Geometry check sheet. Reference: the model listing, model coordinates, mm. A direction names the side the tool comes from. Round coordinates to 2 decimals unless told otherwise and drop trailing zeros. Write each loop counter-clockwise with the first axis right and the second up, starting at its lowest first coordinate (ties: lowest second). Pieces come first, ordered by that corner, then holes. Notation, with made-up numbers: (67, 86) -> (115, 86) arc R25 ccw to (115, 121) -> close; hole circle Ø3 at (-16, 69). An arc over 180 degrees is marked (long way). One line per question, with ' | ' between items.
```python
from build123d import *

# Parameters (mm, degrees)
SKETCH2_R                = 7
BOSS_EXTRUDE1_DEPTH      = 20
BOSS_EXTRUDE1_2_DEPTH    = 20
BOSS_EXTRUDE4_DEPTH      = 25
BOSS_EXTRUDE4_DEPTH_BACK = 25
BOSS_EXTRUDE5_REACH      = 52
SKETCH5_W                = 40
SKETCH5_H                = 30
SKETCH5_W_2              = 30
SKETCH5_H_2              = 20
SKETCH6_R                = 7.5
CUT_EXTRUDE1_DEPTH       = 51


with BuildPart() as part:
    # Sketch2 → Boss-Extrude1 (new body)
    with BuildSketch(Plane(origin=(0, 0, 0), x_dir=(1, 0, 0), z_dir=(0, 1, 0))):
        with BuildLine():
            Line((-55, 15), (-35, 15))
            Line((-35, 15), (-35, -15))
            Line((-35, -15), (-55, -15))
            ThreePointArc((-55, -15), (-70, 0), (-55, 15))
        make_face()
        with Locations((-55, 0)):
            Circle(SKETCH2_R, mode=Mode.SUBTRACT)
    extrude(amount=BOSS_EXTRUDE1_DEPTH)



with BuildPart() as body_2:
    # Sketch2 → Boss-Extrude1 2 (new body)
    with BuildSketch(Plane(origin=(0, 0, 0), x_dir=(1, 0, 0), z_dir=(0, 1, 0))):
        with BuildLine():
            Line((35, -15), (55, -15))
            ThreePointArc((55, -15), (70, 0), (55, 15))
            Line((55, 15), (35, 15))
            Line((35, 15), (35, -15))
        make_face()
        with Locations((55, 0)):
            Circle(SKETCH2_R, mode=Mode.SUBTRACT)
    extrude(amount=BOSS_EXTRUDE1_2_DEPTH)


with BuildPart() as part_1:
    add(part.part)

    add(body_2.part)  # Boss-Extrude4 merges body 2
    # Sketch3 → Boss-Extrude4 (add, two sides)
    with BuildSketch(Plane.XY) as boss_extrude4_sk:
        with BuildLine():
            ThreePointArc((29.580398915, 5), (0, 30), (-29.580398915, 5))
            Line((-29.580398915, 5), (-35, 5))
            Line((-35, 5), (-35, 0))
            Line((-35, 0), (-40, 0))
            ThreePointArc((-40, 0), (0, 40), (40, 0))
            Line((40, 0), (35, 0))
            Line((35, 0), (35, 5))
            Line((35, 5), (29.580398915, 5))
        make_face()
    extrude(amount=BOSS_EXTRUDE4_DEPTH)
    extrude(boss_extrude4_sk.sketch, amount=-BOSS_EXTRUDE4_DEPTH_BACK)

    # Sketch5 → Boss-Extrude5 (add, up to next)
    with BuildSketch(Plane(origin=(0, 50, 0), x_dir=(1, 0, 0), z_dir=(0, 1, 0)), mode=Mode.PRIVATE) as boss_extrude5_sk1:
        Rectangle(SKETCH5_W, SKETCH5_H)
        Rectangle(SKETCH5_W_2, SKETCH5_H_2, mode=Mode.SUBTRACT)
    boss_extrude5_tool1 = extrude(boss_extrude5_sk1.sketch, amount=-BOSS_EXTRUDE5_REACH, mode=Mode.PRIVATE) - part_1.part
    add(boss_extrude5_tool1.solids().sort_by_distance((0, 50, 14.5))[0])

    # Sketch6 → Cut-Extrude1 (cut, through all)
    with BuildSketch(Plane(origin=(0, 50, 0), x_dir=(1, 0, 0), z_dir=(0, 1, 0))):
        Circle(SKETCH6_R)
    extrude(amount=-CUT_EXTRUDE1_DEPTH, mode=Mode.SUBTRACT)


solid = part_1.part
```
(1) Go/stop test with flat-tipped pins: pin 1 (5 mm diameter, centred on x = -45.5, z = -7.5, fed in from -Y); pin 2 (6 mm diameter, centred on x = -43.5, y = 7, fed in from -Z); pin 3 (7.5 mm diameter, centred on y = 39.5, z = 6.5, fed in from +X); pin 4 (6 mm diameter, centred on y = 41.5, z = 2, fed in from -X). Record where each tip stops, or that it passes through.
Resolved:
pin 1: stops at y = 0 | pin 2: stops at z = -15 | pin 3: stops at x = 20 | pin 4: stops at x = -20
(2) Material ranges on line 1 (Z direction, x = 0, y = 35.25); line 2 (Z direction, x = -55, y = 13.75); line 3 (X direction, y = 37, z = 0), recorded low to high.
Resolved:
line 1: z = -25 to -7.5, 7.5 to 25 | line 2: z = -15 to -7, 7 to 15 | line 3: x = -20 to -7.5, 7.5 to 20
(3) Sectioned sample at A-A on x = 0. Record the cut outline in (y, z).
Resolved:
outline: (30, -25) -> (40, -25) -> (40, -15) -> (50, -15) -> (50, -10) -> (40, -10) -> (40, -7.5) -> (30, -7.5) -> close; (30, 7.5) -> (40, 7.5) -> (40, 10) -> (50, 10) -> (50, 15) -> (40, 15) -> (40, 25) -> (30, 25) -> close
(4) Access from +Z, -Z, +X, -X, +Y, -Y to the whole of each face (thin tool, end or side, straight path). Record for faces 1 (the flat face through (0, 45, -10)), 2 (the flat face through (-48, 20, -4)), 3 (the flat face through (0.2, 30.5, -25)), 4 (the flat face through (32, 5, 0)).
Resolved:
face 1: +Y | face 2: +Z, -Z, -X, +Y | face 3: -Z, +X, -X, +Y, -Y | face 4: +Z, -Z, -Y
(5) Sectioned sample at D-D on y = 25. Record the cut outline in (x, z).
Resolved:
outline: (-31.22, -25) -> (-16.58, -25) -> (-16.58, 25) -> (-31.22, 25) -> close; (16.58, -25) -> (31.22, -25) -> (31.22, 25) -> (16.58, 25) -> close
(6) Sectioned sample at C-C on z = 0. Count the separate pieces of the cut face and the enclosed holes in it, then the cut area to 3 significant figures.
Resolved:
separate pieces: 4 | enclosed holes: 0 | area: 1,750 mm2
(7) Sectioned sample at B-B on y = 18. Record the cut outline in (x, z), then the cut area to 3 significant figures.
Resolved:
outline: (-55, -15) -> (-35.72, -15) -> (-35.72, -25) -> (-24, -25) -> (-24, 25) -> (-35.72, 25) -> (-35.72, 15) -> (-55, 15) arc R15 ccw to start; (24, -25) -> (35.72, -25) -> (35.72, -15) -> (55, -15) arc R15 ccw to (55, 15) -> (35.72, 15) -> (35.72, 25) -> (24, 25) -> close; hole circle Ø14 at (-55, 0); hole circle Ø14 at (55, 0) | area: 2,730 mm2
